Build history of the part. All positions in model axes, mm. A direction names the side the tool comes from. Round coordinates to 2 decimals unless told otherwise and drop trailing zeros. Write each loop counter-clockwise with the first axis right and the second up, starting at its lowest first coordinate (ties: lowest second). Pieces come first, ordered by that corner, then holes. Notation, with made-up numbers: (43, 11.25) -> (99, 11.25) arc R17 ccw to (99, 36.25) -> close; hole circle Ø11 at (86.25, -25). An arc over 180 degrees is marked (long way). Answer as CSV lines item,"result".
from build123d import *

# Parameters (mm, degrees)
SKETCH1_R                         = 2.7
BOSS_EXTRUDE1_DEPTH               = 18.5
CUT_EXTRUDE1_DEPTH                = 8
SKETCH3_R                         = 1
CUT_EXTRUDE2_DEPTH                = 6
CORTAR_EXTRUIR1_REACH             = 21.242
CORTAR_EXTRUIR1_DIRECTION_2_REACH = 21.242


with BuildPart() as part:
    # Sketch1 → Boss-Extrude1 (new, symmetric)
    with BuildSketch(Plane(origin=(0, 0, 0), x_dir=(0, 0, -1), z_dir=(1, 0, 0))):
        Circle(SKETCH1_R)
    extrude(amount=BOSS_EXTRUDE1_DEPTH, both=True)

    # Sketch2 → Cut-Extrude1 (cut)
    with BuildSketch(Plane(origin=(18.5, 0, 0), x_dir=(0, 0, -1), z_dir=(1, 0, 0))):
        with BuildLine():
            Line((-1.85, 1.966596044), (-1.85, -1.966596044))
            ThreePointArc((-1.85, -1.966596044), (-2.7, 0), (-1.85, 1.966596044))
        make_face()
        with BuildLine():
            Line((1.85, 1.966596044), (1.85, -1.966596044))
            ThreePointArc((1.85, -1.966596044), (2.7, 0), (1.85, 1.966596044))
        make_face()
    cut_extrude1 = extrude(amount=-CUT_EXTRUDE1_DEPTH, mode=Mode.SUBTRACT)

    # Sketch3 → Cut-Extrude2 (cut)
    with BuildSketch(Plane(origin=(18.5, 0, 0), x_dir=(0, 0, -1), z_dir=(1, 0, 0))):
        Circle(SKETCH3_R)
    cut_extrude2 = extrude(amount=-CUT_EXTRUDE2_DEPTH, mode=Mode.SUBTRACT)

    # Mirror1: Cut-Extrude1, Cut-Extrude2 across plane
    add(cut_extrude1.mirror(Plane(origin=(0, 0, 0), x_dir=(0, 0, 1), z_dir=(1, 0, 0))), mode=Mode.SUBTRACT)
    add(cut_extrude2.mirror(Plane(origin=(0, 0, 0), x_dir=(0, 0, 1), z_dir=(1, 0, 0))), mode=Mode.SUBTRACT)

    # Croquis1 → Cortar-Extruir1 (cut, up to next)
    with BuildSketch(Plane(origin=(0, 0, -1.85), x_dir=(-1, 0, 0), z_dir=(0, 0, -1)), mode=Mode.PRIVATE) as cortar_extruir1_sk1:
        Polygon((-9.5, -2.7), (-9.5, 3.118496514), (-19.119942129, 3.118496514), (-19.119942129, -3.62450436), (-9.5, -3.62450436), align=None)
    cortar_extruir1_tool1 = extrude(cortar_extruir1_sk1.sketch, amount=-CORTAR_EXTRUIR1_REACH, mode=Mode.PRIVATE) & part.part
    add(cortar_extruir1_tool1.solids().sort_by_distance((14.309971, -0.253004, -1.85))[0], mode=Mode.SUBTRACT)

    # Croquis1 → Cortar-Extruir1 direction 2 (cut, up to next)
    with BuildSketch(Plane(origin=(0, 0, -1.85), x_dir=(-1, 0, 0), z_dir=(0, 0, -1)), mode=Mode.PRIVATE) as cortar_extruir1_direction_2_sk1:
        Polygon((-9.5, -2.7), (-9.5, 3.118496514), (-19.119942129, 3.118496514), (-19.119942129, -3.62450436), (-9.5, -3.62450436), align=None)
    cortar_extruir1_direction_2_tool1 = extrude(cortar_extruir1_direction_2_sk1.sketch, amount=CORTAR_EXTRUIR1_DIRECTION_2_REACH, mode=Mode.PRIVATE) & part.part
    add(cortar_extruir1_direction_2_tool1.solids().sort_by_distance((14.309971, -0.253004, -1.85))[0], mode=Mode.SUBTRACT)


solid = part.part
1. Cut at B-B, the plane y = 0. Write the cut outline in (x, z).
Results found:
outline,"(-18.5, -1.85) -> (-10.5, -1.85) -> (-10.5, -2.7) -> (9.5, -2.7) -> (9.5, 2.7) -> (-10.5, 2.7) -> (-10.5, 1.85) -> (-18.5, 1.85) -> (-18.5, 1) -> (-12.5, 1) -> (-12.5, -1) -> (-18.5, -1) -> close"
2. Mould opens along Y. For faces 1 (the cylindrical face through (-1.193, -1.034, -2.494)), 2 (the flat face through (-18.5, -1, 1)), 3 (the cylindrical face through (-16, -1, 0)) say: +Y half, -Y half, draft (parallel to the pull), parting line (faces both ways), or undercut.
Results found:
face 1,"parting line"
face 2,"draft"
face 3,"undercut"
3. Cut at D-D, the plane y = 1.7. Write the cut outline in (x, z).
Results found:
outline,"(-18.5, -1.85) -> (-10.5, -1.85) -> (-10.5, -2.1) -> (9.5, -2.1) -> (9.5, 2.1) -> (-10.5, 2.1) -> (-10.5, 1.85) -> (-18.5, 1.85) -> close"
4. Probe line 1 along Y through (x, z) = (-14, 0); line 2 along Y through (x, z) = (-16, -0.5); line 3 along X through (y, z) = (-0.1, 0). List the from-to ranges inside material, lowest first.
Results found:
line 1,"y = -2.7 to -1, 1 to 2.7"
line 2,"y = -2.65 to -0.87, 0.87 to 2.65"
line 3,"x = -12.5 to 9.5"
5. Cut at C-C, the plane x = -12.25. Write the cut outline in (y, z).
Results found:
outline,"(-1.97, -1.85) -> (1.97, -1.85) arc R2.7 ccw to (1.97, 1.85) -> (-1.97, 1.85) arc R2.7 ccw to start"
6. Drop flat-ended pins along their axis: pin 1 Ø1 at (x, y) = (-9.5, -0.5) entering from +Z; pin 2 Ø2 at (x, y) = (-8.5, 1.5) entering from -Z; pin 3 Ø1.2 at (x, y) = (-14.5, -0.5) entering from +Z; pin 4 Ø1.5 at (x, y) = (2.5, -2) entering from +Z. Give the stop position or say it passes through.
Results found:
pin 1,"stops at z = 2.7"
pin 2,"stops at z = -2.65"
pin 3,"stops at z = 1.85"
pin 4,"stops at z = 2.39"
7. Which spindle directions (+Z, -Z, +X, -X, +Y, -Y) get a long thin tool onto all of the face, cutting with end or side? Do faces 4 (the flat face through (-15, 0, 1.85)), 5 (the flat face through (-15, 0, -1.85)), 6 (the flat face through (9.5, 0, 0)), 7 (the flat face through (-12.5, 0, 0)). Say none if no direction does.
Results found:
face 4,"+Z, -X, +Y, -Y"
face 5,"-Z, -X, +Y, -Y"
face 6,"+Z, -Z, +X, +Y, -Y"
face 7,"-X"
8. Cut at A-A, the plane z = 0. Write the cut outline in (x, y), then the cut area to 3 significant figures.
Results found:
outline,"(-18.5, -2.7) -> (9.5, -2.7) -> (9.5, 2.7) -> (-18.5, 2.7) -> (-18.5, 1) -> (-12.5, 1) -> (-12.5, -1) -> (-18.5, -1) -> close"
area,"139 mm2"
